CAD build for the part. Positions are in the model's coordinates, mm. Coordinates: 2 decimals unless noted, no trailing zeros. Write each loop counter-clockwise with the first axis right and the second up, starting at its lowest first coordinate (ties: lowest second). Pieces come first, ordered by that corner, then holes. Notation, with made-up numbers: (2, 11.25) - (19, 11.25) arc R18 ccw to (19, 34.25) - close; hole circle Ø9 at (-22, -5). An arc over 180 degrees is marked (long way). Answer in a Markdown table with one row per item. Add a question column.
Q1. Drill centre lines: line 1 along X through (y, z) = (-1.5, 0.75); line 2 along X through (y, z) = (-4.75, 0.2); line 3 along X through (y, z) = (7.5, 0.55). Where is each one in solid material? Low to high. Write a range as from..to.
Q2. Band-saw the part on D-D (x = 6). List the corners of the cut face in (y, z).
Q3. Band-saw the part on C-C (y = 1.25). List the corners of the cut face in (x, z).
Q4. Band-saw the part on A-A (y = -8.25). List the corners of the cut face in (x, z).
Q5. Band-saw the part on B-B (z = 0.8). List the corners of the cut face in (x, y), and give its area (3 significant figures).
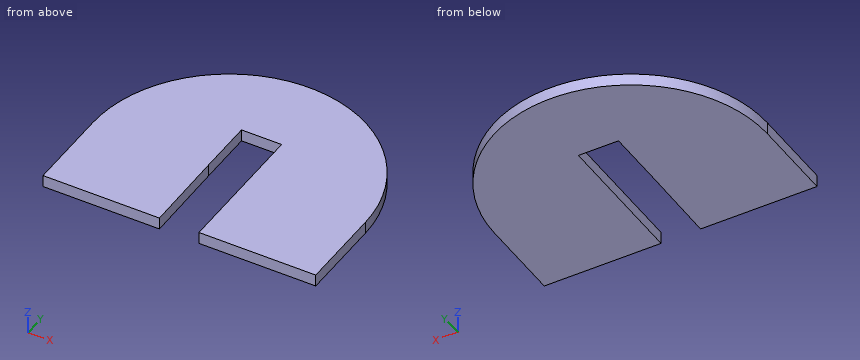
```python
from build123d import *

# Parameters (mm, degrees)
F1_DEPTH = 1.5


with BuildPart() as f1:
    # F0 (on Top) → F1 (new body)
    with BuildSketch(Plane.XY):
        with BuildLine():
            Line((17.480557, -15.692959), (17.480557, -5.109434))
            ThreePointArc((17.480557, -5.109434), (0.480557, 11.890566), (-16.519443, -5.109434))
            Line((-16.519443, -5.109434), (-16.519443, -15.692959))
            Line((-16.519443, -15.692959), (-2.00486, -15.692959))
            Line((-2.00486, -15.692959), (-2.081214, -5.109434))
            Line((-2.081214, -5.109434), (-2.081214, 1.907042))
            Line((-2.081214, 1.907042), (0.418786, 1.907042))
            Line((0.418786, 1.907042), (2.918786, 1.907042))
            Line((2.918786, 1.907042), (2.918786, -5.109434))
            Line((2.918786, -5.109434), (2.918786, -15.692959))
            Line((2.918786, -15.692959), (17.480557, -15.692959))
        make_face()
    extrude(amount=F1_DEPTH)


solid = f1.part
```
Checked values:
| question | item | result |
|---|---|---|
| 1 | line 1 | x = -16.13..-2.08, 2.92..17.09 |
| 1 | line 2 | x = -16.52..-2.08, 2.92..17.48 |
| 1 | line 3 | x = -10.92..11.88 |
| 2 | outline | (-15.69, 0) - (10.97, 0) - (10.97, 1.5) - (-15.69, 1.5) - close |
| 3 | outline | (-15.29, 0) - (-2.08, 0) - (-2.08, 1.5) - (-15.29, 1.5) - close; (2.92, 0) - (16.25, 0) - (16.25, 1.5) - (2.92, 1.5) - close |
| 4 | outline | (-16.52, 0) - (-2.06, 0) - (-2.06, 1.5) - (-16.52, 1.5) - close; (2.92, 0) - (17.48, 0) - (17.48, 1.5) - (2.92, 1.5) - close |
| 5 | outline | (-16.52, -15.69) - (-2, -15.69) - (-2.08, -5.11) - (-2.08, 1.91) - (2.92, 1.91) - (2.92, -15.69) - (17.48, -15.69) - (17.48, -5.11) arc R17 ccw to (-16.52, -5.11) - close |
| 5 | area | 726 mm² |
